Design review of the part built by this model. Coordinates are the model's own, in mm. A direction names the side the tool comes from. Give positions to 0.01 mm unless a question says otherwise; leave off trailing zeros. Order: outer loops, then holes, each group sorted by start corner. A loop starts at its lowest first (then second) coordinate and runs counter-clockwise, first axis right, second up. Notation, with made-up numbers: (-15.5, 29.25) -> (29.5, 29.25) arc R24 ccw to (29.5, 41.25) -> close; hole circle Ø10 at (30, 82.5). An arc over 180 degrees is marked (long way). One line per item, written item: value. Start each with the question number.
1) Consider section C-C (z = 53). State the section outline as (x, y) points, plus the area to 3 significant figures.
2) Tool access review of faces 4 (the face through (32.68, 10.29, 45.51)), 5 (the face through (-9.703, -43.694, 24.783)): name each direction out of +Z, -Z, +X, -X, +Y, -Y from which nothing blocks a thin tool from reaching the whole face with its end or side.
3) Wall thickness on line 1 along Z through (x, y) = (28.5, 26); line 2 along Y through (x, z) = (18, 117.5); line 3 along X through (y, z) = (13, 88.5): over which ranges is each line inside the solid? List them lowest first. Write a range as from..to.
4) For pin 1 (1.5 mm diameter, centred on y = -14, z = 94.5, fed in from -X); pin 2 (1 mm diameter, centred on x = -34.5, z = 69.5, fed in from -Y); pin 3 (5 mm diameter, centred on y = 27, z = 99, fed in from +X), all flat-tipped, find the tip position at first contact; note any pin that passes through.
5) Consider section B-B (z = 22). State the section outline as (x, y) points, plus the area to 3 significant figures.
6) Consider section A-A (x = 0). State the section outline as (y, z) points.
7) The part is to be moulded in two halves that separate along Z. For faces 1 (the face through (0, 0, 154.94)), 2 (the face through (-9.72, -43.78, 0.79)), 3 (the face through (-30, 11, 25.4)), say which applies: released by +Z, released by -Z, zero draft, split by the parting line, or undercut.
from build123d import *

# Parameters (mm, degrees)
F0_R       = 44.45
F2_R       = 50.8
F3_FACE_R  = 50.8
F5_R       = 44.45
F7_R       = 31.75
F9_R       = 38.1
F10_FACE_R = 38.1
F12_R      = 31.75


with BuildPart() as f3:
    # F0 (on Top) → F3 section 0
    with BuildSketch(Plane.XY):
        Circle(F0_R)
    # F2 (on offset) → F3 section 1
    with BuildSketch(Plane.XY.offset(12.7)):
        Circle(F2_R)
    loft()

    # F3_face (on face) → F6 section 0
    with BuildSketch(Plane.XY.offset(12.7)):
        Circle(F3_FACE_R)
    # F5 (on offset) → F6 section 1
    with BuildSketch(Plane.XY.offset(25.4)):
        Circle(F5_R)
    loft()

    # F7 (on offset) → F10 section 0
    with BuildSketch(Plane.XY.offset(25.4)):
        Circle(F7_R)
    # F9 (on offset) → F10 section 1
    with BuildSketch(Plane.XY.offset(76.2)):
        Circle(F9_R)
    loft()

    # F10_face (on face) → F13 section 0
    with BuildSketch(Plane.XY.offset(76.2)):
        Circle(F10_FACE_R)
    # F12 (on offset) → F13 section 1
    with BuildSketch(Plane.XY.offset(154.94)):
        Circle(F12_R)
    loft()


solid = f3.part
Checked values:
1. outline: circle Ø70.4 at (0, 0)
1. area: 3,890 mm^2
2. face 4: none
2. face 5: +Z
3. line 1: z = 0..25.4
3. line 2: y = -29.75..29.75
3. line 3: x = -34.76..34.76
4. pin 1: stops at x = -34.15
4. pin 2: stops at y = -15.26
4. pin 3: stops at x = 26.75
5. outline: circle Ø92.3 at (0, 0)
5. area: 6,690 mm^2
6. outline: (-50.8, 12.7) -> (-44.45, 0) -> (44.45, 0) -> (50.8, 12.7) -> (44.45, 25.4) -> (31.75, 25.4) -> (38.1, 76.2) -> (31.75, 154.94) -> (-31.75, 154.94) -> (-38.1, 76.2) -> (-31.75, 25.4) -> (-44.45, 25.4) -> close
7. face 1: released by +Z
7. face 2: released by -Z
7. face 3: undercut
